Source: CAD feature listing. Evaluate the final solid. Frame: model axes, mm. Face numbers are marked on the shaded views. A direction names the side the tool comes from. Round coordinates to 2 decimals unless told otherwise and drop trailing zeros. Loops run counter-clockwise (first coordinate to the right, second up) from the corner with the lowest first, then second, coordinate; pieces in that order, holes last. Notation, with made-up numbers: M 33.5,12 L 60.5,12 A22 ccw 60.5,47 Z; hole C 23.25,43.25 d6. An arc over 180 degrees is marked long. Answer as a JSON object with one key per item and string values.
from build123d import *

# Parameters (mm, degrees)
ESQUISSE1_R                  = 2.8
BASE_EXTRUSION_DEPTH         = 1.8
CONG_1_R                     = 0.8
ESQUISSE2_R                  = 1.5
BOSS_EXTRU_1_DEPTH           = 6
CHANFREIN1_SIZE              = 0.2
ESQUISSE3_W                  = 1
ESQUISSE3_H                  = 1
ENL_V_MAT_EXTRU_1_DEPTH      = 3.8000001
ENL_V_MAT_EXTRU_1_DEPTH_BACK = 3.8


with BuildPart() as part:
    # Esquisse1 → Base-Extrusion (new body)
    with BuildSketch(Plane.XY):
        Circle(ESQUISSE1_R)
    extrude(amount=BASE_EXTRUSION_DEPTH)

    # Cong_1
    cong_1_edges = [part.edges().sort_by_distance(p)[0] for p in [
        (-2.8, 0, 0),
    ]]
    fillet(cong_1_edges, radius=CONG_1_R)

    # Esquisse2 → Boss.-Extru.1 (add)
    with BuildSketch(Plane.XY.offset(1.8)):
        Circle(ESQUISSE2_R)
    extrude(amount=BOSS_EXTRU_1_DEPTH)

    # Chanfrein1
    chanfrein1_edges = [part.edges().sort_by_distance(p)[0] for p in [
        (-1.5, 0, 7.8),
    ]]
    chamfer(chanfrein1_edges, length=CHANFREIN1_SIZE)

    # Esquisse3 → Enl_v. mat.-Extru.1 (cut, two sides)
    with BuildSketch(Plane(origin=(0, 0, 0), x_dir=(1, 0, 0), z_dir=(0, 1, 0))) as enl_v_mat_extru_1_sk:
        with Locations((0, -0.5)):
            Rectangle(ESQUISSE3_W, ESQUISSE3_H)
    extrude(amount=ENL_V_MAT_EXTRU_1_DEPTH, mode=Mode.SUBTRACT)
    extrude(enl_v_mat_extru_1_sk.sketch, amount=-ENL_V_MAT_EXTRU_1_DEPTH_BACK, mode=Mode.SUBTRACT)


solid = part.part
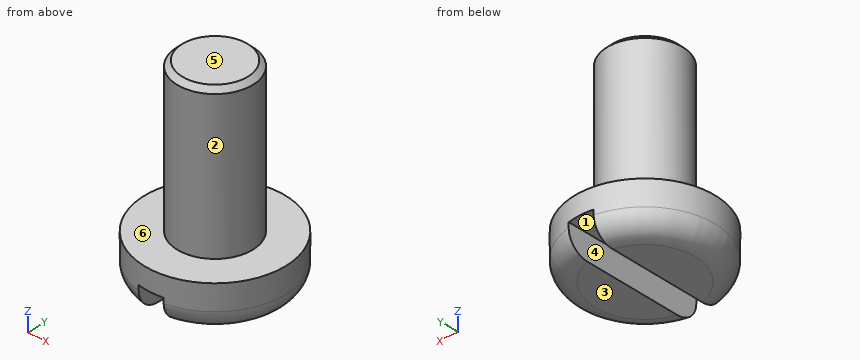
Item 1: Section B-B on x = 0. Return the cut outline in (y, z).
Answer sheet:
{"outline": "M -2.8,1 L 2.8,1 L 2.8,1.8 L 1.5,1.8 L 1.5,7.6 L 1.3,7.8 L -1.3,7.8 L -1.5,7.6 L -1.5,1.8 L -2.8,1.8 Z"}
Item 2: Access query for the marked faces 5 and 6. Directions: +Z, -Z, +X, -X, +Y, -Y. A direction counts if a zero-diameter tool reaches every point of the face in a straight line with its end or side. Return the directions, or none.
Answer sheet:
{"face 5": "+Z, +X, -X, +Y, -Y", "face 6": "+Z"}
Item 3: Section C-C on z = 1.5. Return the cut outline in (x, y), then the cut area to 3 significant figures.
Answer sheet:
{"outline": "C 0,0 d5.6", "area": "24.6 mm²"}
Item 4: Section A-A on y = 0. Return the cut outline in (x, z), then the cut area to 3 significant figures.
Answer sheet:
{"outline": "M -2.8,0.8 A0.8 ccw -2,0 L -0.5,0 L -0.5,1 L 0.5,1 L 0.5,0 L 2,0 A0.8 ccw 2.8,0.8 L 2.8,1.8 L 1.5,1.8 L 1.5,7.6 L 1.3,7.8 L -1.3,7.8 L -1.5,7.6 L -1.5,1.8 L -2.8,1.8 Z", "area": "26.8 mm²"}
Item 5: Pull-direction query (X, two-part tool) for the marked faces 1, 2, 3 and 4; classes: pulls with the +X half, pulls with the -X half, needs draft (parallel to the pull), parting line crosses it, or undercut.
Answer sheet:
{"face 1": "undercut", "face 2": "parting line crosses it", "face 3": "needs draft", "face 4": "undercut"}
Item 6: Line query: probe 1 along X at (y, z) = (0.75, 6.25); probe 2 along Z at (x, y) = (-2, -0.2); probe 3 along Z at (x, y) = (0.4, 2.4). Output: solid intervals per line, ascending. Write a range as from..to.
Answer sheet:
{"probe 1": "x = -1.3..1.3", "probe 2": "z = 0..1.8", "probe 3": "z = 1..1.8"}
Item 7: Contact query for flat-ended pins moving along their axis: pin 1 Ø1.5 at (y, z) = (-1, 5.5) entering from -X; pin 2 Ø0.5 at (y, z) = (-1, 0.5) entering from -X; pin 3 Ø0.8 at (x, y) = (0, 1) entering from -Z. Output: stop coordinate, or through.
Answer sheet:
{"pin 1": "stops at x = -1.48", "pin 2": "stops at x = -2.67", "pin 3": "stops at z = 1"}
